Part print with two shaded views. Sizes in mm from the minimum x, y, z corner. A direction names the side the tool comes from. Round coordinates to 2 decimals unless told otherwise and drop trailing zeros. Order: outer loops, then holes, each group sorted by start corner. A loop starts at its lowest first (then second) coordinate and runs counter-clockwise, first axis right, second up. Notation, with made-up numbers: M 85.5,29.25 L 104.5,29.25 A10 ccw 104.5,33.25 Z; hole C 50,-22 d2. An arc over 180 degrees is marked long. One line per question, with ' | ' between items.
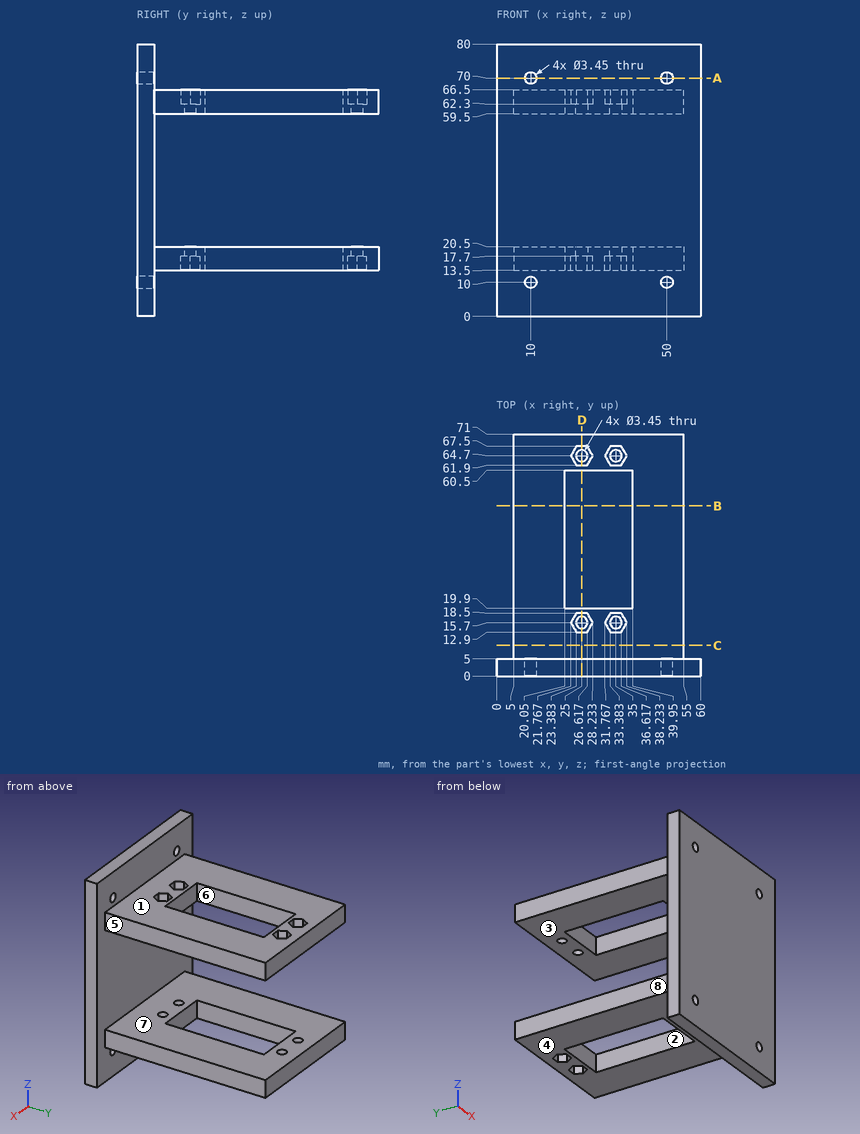
1) Drop flat-ended pins along their axis: pin 1 (1 mm diameter, centred on x = 24, z = 16.5, fed in from -Y); pin 2 (3 mm diameter, centred on x = 34.5, y = 63.5, fed in from +Z); pin 3 (5.5 mm diameter, centred on y = 24, z = 15.5, fed in from -X); pin 4 (5.5 mm diameter, centred on x = 35, y = 15.7, fed in from -Z). Give the stop position or say it passes through.
The answers:
pin 1: stops at y = 0 | pin 2: stops at z = 62.3 | pin 3: stops at x = 5 | pin 4: stops at z = 17.7
2) Which spindle directions (+Z, -Z, +X, -X, +Y, -Y) get a long thin tool onto all of the face, cutting with end or side? Do the marked faces 4, 5, 6, 7 and 8. Say none if no direction does.
The answers:
face 4: -Z, +X, -X, +Y | face 5: +Z, -Z, +X, +Y | face 6: +Z, -Z | face 7: +X, -X, +Y | face 8: +Z, -Z, -X, +Y
3) Saw through at C-C (y = 9). List the corners of the cut face in (x, z).
The answers:
outline: M 5,13.5 L 55,13.5 L 55,20.5 L 5,20.5 Z; M 5,59.5 L 55,59.5 L 55,66.5 L 5,66.5 Z
4) Saw through at A-A (z = 70). List the corners of the cut face in (x, y) (1 decimal).
The answers:
outline: M 0,0 L 8.3,0 L 8.3,5 L 0,5 Z; M 11.7,0 L 48.3,0 L 48.3,5 L 11.7,5 Z; M 51.7,0 L 60,0 L 60,5 L 51.7,5 Z
5) Probe line 1 (Y direction, x = 25, z = 19) (1 decimal); line 2 (X direction, y = 43.5, z = 19); line 3 (X direction, y = 64.7, z = 60.6) (1 decimal). List the from-to ranges inside material, lowest first. Write a range as [from, to].
The answers:
line 1: y = [0, 14], [17.4, 19.9], [60.5, 63], [66.4, 71] | line 2: x = [5, 20.05], [39.95, 55] | line 3: x = [5, 23.3], [26.7, 33.3], [36.7, 55]
6) Saw through at B-B (y = 50). List the corners of the cut face in (x, z).
The answers:
outline: M 5,13.5 L 20.05,13.5 L 20.05,20.5 L 5,20.5 Z; M 5,59.5 L 20.05,59.5 L 20.05,66.5 L 5,66.5 Z; M 39.95,13.5 L 55,13.5 L 55,20.5 L 39.95,20.5 Z; M 39.95,59.5 L 55,59.5 L 55,66.5 L 39.95,66.5 Z
7) Two-plate mould, pull along Z, no slides. Class the marked faces 1, 2 and 3: released by +Z, released by -Z, zero draft, split by the parting line, or undercut.
The answers:
face 1: released by +Z | face 2: zero draft | face 3: undercut
8) Saw through at D-D (x = 25). Give the number of separate pieces and of enclosed holes in the cut face, plus the area to 3 significant figures.
The answers:
separate pieces: 7 | enclosed holes: 0 | area: 623 mm²
